Design review of the part shown in the three views and the two pictorial views. Dimensions are in mm from the part's minimum x, y and z. Give positions to 0.01 mm unless a question says otherwise; leave off trailing zeros. Order: outer loops, then holes, each group sorted by start corner. A loop starts at its lowest first (then second) coordinate and runs counter-clockwise, first axis right, second up.
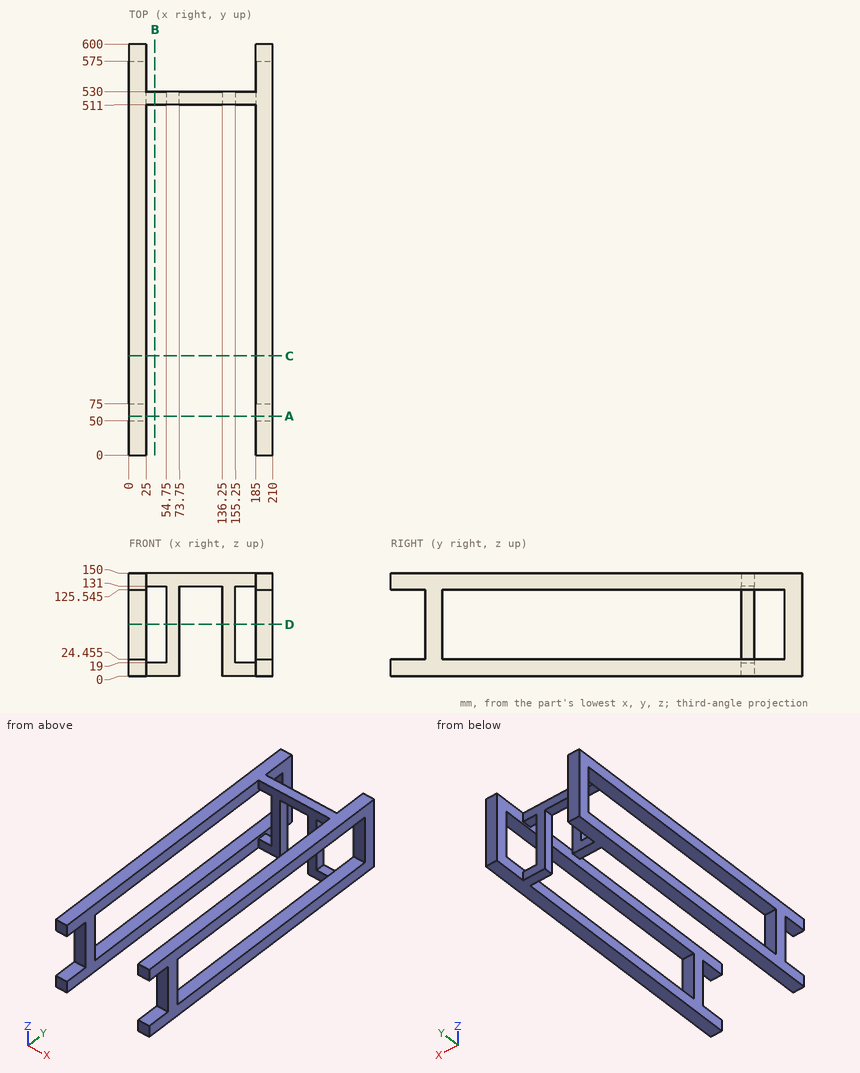
Item 1: Take a section at C-C (y = 145). Give the boundary of the cut face in (x, z) (1 decimal).
Values found:
outline: (0, 0) - (25, 0) - (25, 24.5) - (0, 24.5) - close; (0, 125.5) - (25, 125.5) - (25, 150) - (0, 150) - close; (185, 0) - (210, 0) - (210, 24.5) - (185, 24.5) - close; (185, 125.5) - (210, 125.5) - (210, 150) - (185, 150) - close
Item 2: Take a section at B-B (x = 38). Give the boundary of the cut face in (y, z).
Values found:
outline: (511, 0) - (530, 0) - (530, 19) - (511, 19) - close; (511, 131) - (530, 131) - (530, 150) - (511, 150) - close
Item 3: Take a section at A-A (y = 57). Give the boundary of the cut face in (x, z).
Values found:
outline: (0, 0) - (25, 0) - (25, 150) - (0, 150) - close; (185, 0) - (210, 0) - (210, 150) - (185, 150) - close
Item 4: Clearance check with flat-ended pins moving along their axes: pin 1 Ø7.5 at (x, z) = (196, 99.5) entering from -Y; pin 2 Ø15 at (y, z) = (525, 71) entering from +X; pin 3 Ø10 at (x, z) = (136, 99.5) entering from -Y. State where each tip first meets the part, or that it passes through.
Values found:
pin 1: stops at y = 50
pin 2: stops at x = 155.25
pin 3: stops at y = 511
Item 5: Take a section at D-D (z = 75.5). Give the boundary of the cut face in (x, y).
Values found:
outline: (0, 50) - (25, 50) - (25, 75) - (0, 75) - close; (0, 575) - (25, 575) - (25, 600) - (0, 600) - close; (54.75, 511) - (73.75, 511) - (73.75, 530) - (54.75, 530) - close; (136.25, 511) - (155.25, 511) - (155.25, 530) - (136.25, 530) - close; (185, 50) - (210, 50) - (210, 75) - (185, 75) - close; (185, 575) - (210, 575) - (210, 600) - (185, 600) - close
Item 6: For line 1 (X direction, y = 49, z = 137.5); line 2 (Z direction, x = 199, y = 145.5) (1 decimal); line 3 (Y direction, x = 9.5, z = 40), list the stretches that pass through material, from the lowest coordinate up.
Values found:
line 1: x = 0 to 25, 185 to 210
line 2: z = 0 to 24.5, 125.5 to 150
line 3: y = 50 to 75, 575 to 600
